Autodesk Inventor part; units mm, degrees
ref_plane "YZ Plane" through (0, 0, 0) normal (1, 0, 0) x (0, 1, 0)
ref_plane "XZ Plane" through (0, 0, 0) normal (0, 1, 0) x (-1, 0, 0)
ref_plane "XY Plane" through (0, 0, 0) normal (0, 0, 1) x (1, 0, 0)
sketch "Sketch1" plane through (0, 0, 0) normal (0, 0, 1) x (1, 0, 0)
  line L0 (-12.7, -12.7) -> (12.7, -12.7)
  line L1 (12.7, -12.7) -> (12.7, 12.7)
  line L2 (12.7, 12.7) -> (-12.7, 12.7)
  line L3 (-12.7, 12.7) -> (-12.7, -12.7)
  line L4 (-12.7, -12.7) -> (12.7, 12.7) construction
  line L5 (12.7, -12.7) -> (-12.7, 12.7) construction
  line L6 (-9.525, -9.525) -> (9.525, -9.525)
  line L7 (9.525, -9.525) -> (9.525, 9.525)
  line L8 (9.525, 9.525) -> (-9.525, 9.525)
  line L9 (-9.525, 9.525) -> (-9.525, -9.525)
  line L10 (-9.525, -9.525) -> (9.525, 9.525) construction
  line L11 (9.525, -9.525) -> (-9.525, 9.525) construction
  point P0 (0, 0)
  dimension "d0" = 25.4
  dimension "d1" = 25.4
  dimension "d2" = 3.175
extrude "Extrusion1" add sketch "Sketch1" along normal blind 762
sketch "Sketch2" plane through (12.7, -12.7, 0) normal (1, 0, 0) x (0, 0, -1)
  line L0 (0, 0) -> (0, 25.4)
  line L1 (0, 25.4) -> (-14.6647, 0)
  line L2 (0, 0) -> (-762, 0)
  line L3 (0, 0) -> (0, 25.4)
  line L4 (-14.6647, 0) -> (0, 0)
  point P0 (0, 12.7)
  dimension "d10" = 60
extrude "Extrusion2" cut sketch "Sketch2" against normal through all
sketch "Sketch3" plane through (12.7, -12.7, 762) normal (1, 0, 0) x (0, 0, -1)
  line L0 (762, 25.4) -> (0, 25.4)
  line L1 (0, 25.4) -> (43.9941, 0)
  line L2 (747.3353, 0) -> (0, 0)
  line L3 (0, 0) -> (0, 25.4)
  line L4 (0, 3.175) -> (0, 22.225)
  line L5 (43.9941, 0) -> (0, 0)
  point P0 (762, 12.7)
  dimension "d7" = 30
extrude "Extrusion3" cut sketch "Sketch3" against normal through all
properties part number "hypotAluminumExtrusion"
Verification items for the finished model (mm, model axes). A direction names the side the tool comes from. Round coordinates to 2 decimals unless told otherwise and drop trailing zeros. Loops run counter-clockwise (first coordinate to the right, second up) from the corner with the lowest first, then second, coordinate; pieces in that order, holes last. Notation, with made-up numbers: (8, -29) - (58, -29) arc R11 cw to (58, -20) - close; hole circle Ø2 at (40.5, -32). An arc over 180 degrees is marked (long way). Answer in a Markdown table with one row per item. Add a question column.
Q1. Release check for a two-part mould opening along Y. For faces 3 (the face through (-12.7, 0, 376)), 4 (the face through (0, 12.7, 376)), 5 (the face through (-11, 0, 740)), 6 (the face through (0, 9.525, 374)) record: pulls with the +Y half, pulls with the -Y half, needs draft (parallel to the pull), parting line crosses it, or undercut.
Q2. Section check C-C on z = 442. Enter the section's corners in (x, y) (3 decimals).
Q3. Gauge pin test, flat end, axial feed: pin 1 (1.5 mm diameter, centred on x = -10, y = 8.5, fed in from +Z). Record the tip position at first contact, or that the pin passes through.
Q4. Tool access check on faces 1 (the face through (0, -9.525, 363)), 2 (the face through (0, -12.7, 361)). Record the directions out of +Z, -Z, +X, -X, +Y, -Y that give a thin tool (end or side, any length) a straight path to the whole face; none if there is none.
Q5. Section check B-B on y = -3.5. Enter the section's corners in (x, z) (3 decimals).
Q6. Material ranges on line 1 (X direction, y = -0.5, z = 619.5) (3 decimals); line 2 (Z direction, x = 5.75, y = 10.25), recorded low to high.
Q7. Section check A-A on x = -3. Enter the section's corners in (y, z) (3 decimals).
Found:
| question | item | result |
|---|---|---|
| 1 | face 3 | needs draft |
| 1 | face 4 | pulls with the +Y half |
| 1 | face 5 | pulls with the -Y half |
| 1 | face 6 | undercut |
| 2 | outline | (-12.7, -12.7) - (12.7, -12.7) - (12.7, 12.7) - (-12.7, 12.7) - close; hole (-9.525, -9.525) - (9.525, -9.525) - (9.525, 9.525) - (-9.525, 9.525) - close |
| 3 | pin 1 | stops at z = 756.02 |
| 4 | face 1 | +Z, -Z |
| 4 | face 2 | +Z, -Z, +X, -X, -Y |
| 5 | outline | (-12.7, 9.353) - (-9.525, 9.353) - (-9.525, 733.941) - (-12.7, 733.941) - close; (9.525, 9.353) - (12.7, 9.353) - (12.7, 733.941) - (9.525, 733.941) - close |
| 6 | line 1 | x = -12.7 to -9.525, 9.525 to 12.7 |
| 6 | line 2 | z = 1.41 to 757.76 |
| 7 | outline | (-12.7, 14.665) - (-9.525, 12.832) - (-9.525, 723.505) - (-12.7, 718.006) - close; (9.525, 1.833) - (12.7, 0) - (12.7, 762) - (9.525, 756.501) - close |
